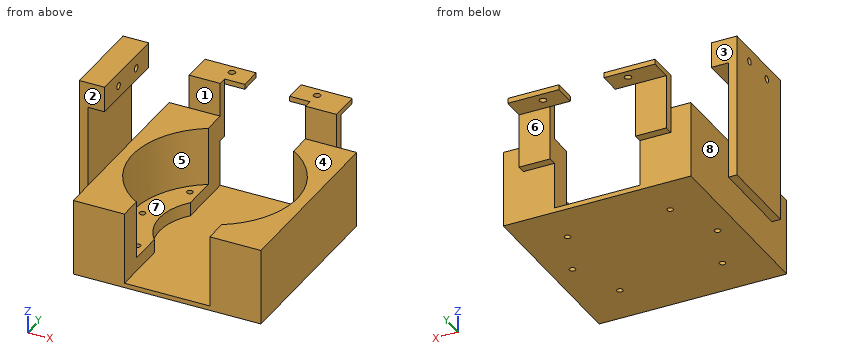
```python
from build123d import *

# Parameters (mm, degrees)
SKETCH_1_W          = 110
SKETCH_1_H          = 110
EXTRUDE_1_DEPTH     = 45
SKETCH_4_R          = 32.5
CUT_EXTRUDE_1_DEPTH = 42.3
SKETCH_5_R          = 48.25
CUT_EXTRUDE_2_DEPTH = 34.3
SKETCH_6_W          = 50
SKETCH_6_H          = 110
CUT_EXTRUDE_3_DEPTH = 8
CUT_EXTRUDE_4_DEPTH = 42.3
SKETCH_8_R          = 1.75
CUT_EXTRUDE_5_DEPTH = 160.3
SKETCH_9_W          = 18.158603558
SKETCH_9_H          = 15
SKETCH_9_H_2        = 20
EXTRUDE_2_DEPTH     = 5
SKETCH_10_W         = 30
SKETCH_10_H         = 3
EXTRUDE_3_DEPTH     = 13
SKETCH_11_R         = 2
CUT_EXTRUDE_6_DEPTH = 168.463428843
SKETCH_12_W         = 85
SKETCH_12_H         = 50
EXTRUDE_4_DEPTH     = 5
EXTRUDE_5_REACH     = 191.262
SKETCH_13_W         = 15
SKETCH_13_H         = 50
CUT_EXTRUDE_8_REACH = 194.211
SKETCH_15_RX        = 2
SKETCH_15_RY        = 1.999994073


with BuildPart() as part:
    # 草图1 → 凸台-拉伸1 (new body)
    with BuildSketch(Plane.XY):
        with Locations((55, -55)):
            Rectangle(SKETCH_1_W, SKETCH_1_H)
    extrude(amount=EXTRUDE_1_DEPTH)

    # 草图4 → 切除-拉伸1 (cut)
    with BuildSketch(Plane.XY.offset(45)):
        with Locations((55, -55)):
            Circle(SKETCH_4_R)
    extrude(amount=-CUT_EXTRUDE_1_DEPTH, mode=Mode.SUBTRACT)

    # 草图5 → 切除-拉伸2 (cut)
    with BuildSketch(Plane.XY.offset(45)):
        with Locations((55, -55)):
            Circle(SKETCH_5_R)
    extrude(amount=-CUT_EXTRUDE_2_DEPTH, mode=Mode.SUBTRACT)

    # 草图6 → 切除-拉伸3 (cut)
    with BuildSketch(Plane.XY.offset(10.7)):
        with Locations((55, -55)):
            Rectangle(SKETCH_6_W, SKETCH_6_H)
    extrude(amount=-CUT_EXTRUDE_3_DEPTH, mode=Mode.SUBTRACT)

    # 草图7 → 切除-拉伸4 (cut)
    with BuildSketch(Plane.XY.offset(45)):
        with BuildLine():
            Line((80, -34.233440343), (80, 0))
            Line((80, 0), (30, 0))
            Line((30, 0), (30, -34.233440343))
            ThreePointArc((30, -34.233440343), (22.5, -55), (30, -75.766559657))
            Line((30, -75.766559657), (30, -110))
            Line((30, -110), (80, -110))
            Line((80, -110), (80, -75.766559657))
            ThreePointArc((80, -75.766559657), (87.5, -55), (80, -34.233440343))
        make_face()
    extrude(amount=-CUT_EXTRUDE_4_DEPTH, mode=Mode.SUBTRACT)

    # 草图8 → 切除-拉伸5 (cut, through all)
    with BuildSketch(Plane.XY.offset(10.7)):
        with Locations((12.5, -55)):
            Circle(SKETCH_8_R)
        with Locations((24.9479618, -24.9479618)):
            Circle(SKETCH_8_R)
        with Locations((85.0520382, -24.9479618)):
            Circle(SKETCH_8_R)
        with Locations((97.5, -55)):
            Circle(SKETCH_8_R)
        with Locations((85.0520382, -85.0520382)):
            Circle(SKETCH_8_R)
        with Locations((24.9479618, -85.0520382)):
            Circle(SKETCH_8_R)
    extrude(amount=-CUT_EXTRUDE_5_DEPTH, mode=Mode.SUBTRACT)

    # 草图9 → 凸台-拉伸2 (add)
    with BuildSketch(Plane(origin=(0, 0, 0), x_dir=(1, 0, 0), z_dir=(0, 1, 0))):
        with Locations((20.920698221, -37.5)):
            Rectangle(SKETCH_9_W, SKETCH_9_H)
        with Locations((20.920698221, -55)):
            Rectangle(SKETCH_9_W, SKETCH_9_H_2)
        with Locations((89.079301779, -37.5)):
            Rectangle(SKETCH_9_W, SKETCH_9_H)
        with Locations((89.079301779, -55)):
            Rectangle(SKETCH_9_W, SKETCH_9_H_2)
    extrude(amount=EXTRUDE_2_DEPTH)

    # 草图10 → 凸台-拉伸3 (add)
    with BuildSketch(Plane(origin=(0, 5, 0), x_dir=(1, 0, 0), z_dir=(0, 1, 0))):
        with Locations((83.158603558, -63.5)):
            Rectangle(SKETCH_10_W, SKETCH_10_H)
        with Locations((26.841396442, -63.5)):
            Rectangle(SKETCH_10_W, SKETCH_10_H)
    extrude(amount=EXTRUDE_3_DEPTH)

    # 草图11 → 切除-拉伸6 (cut, through all)
    with BuildSketch(Plane(origin=(0, 0, 62), x_dir=(-1, 0, 0), z_dir=(0, 0, -1))):
        with Locations((-30.425668719, 12.656132332)):
            Circle(SKETCH_11_R)
        with Locations((-80.424676819, 12.34118954)):
            Circle(SKETCH_11_R)
    extrude(amount=-CUT_EXTRUDE_6_DEPTH, mode=Mode.SUBTRACT)

    # 草图12 → 凸台-拉伸4 (add)
    with BuildSketch(Plane.ZY):
        with Locations((65.296402905, -68.092997568)):
            Rectangle(SKETCH_12_W, SKETCH_12_H)
    extrude(amount=EXTRUDE_4_DEPTH)

    # 凸台-拉伸5: up to this plane
    extrude_5_end = Plane(origin=(9.859168453, -77.216105133, 215), z_dir=(-0.9999801620108199, 0.006298855833765048, 1.0454600148553557e-15))
    # 草图13 → 凸台-拉伸5 (add, up to the surface)
    with BuildSketch(Plane(origin=(0, 0, 0), x_dir=(0, 0, -1), z_dir=(1, 0, 0)), mode=Mode.PRIVATE) as extrude_5_sk1:
        with Locations((-100.296402905, -68.092997568)):
            Rectangle(SKETCH_13_W, SKETCH_13_H)
    extrude_5_tool1 = split(extrude(extrude_5_sk1.sketch, amount=EXTRUDE_5_REACH, mode=Mode.PRIVATE), bisect_by=extrude_5_end, keep=Keep.BOTH, mode=Mode.PRIVATE)
    add(extrude_5_tool1.solids().sort_by_distance((0, -68.092998, 100.296403))[0])

    # 切除-拉伸8: up to this plane
    cut_extrude_8_end = Plane(origin=(9.859168453, -77.216105133, 215), z_dir=(-0.9999801620108199, 0.006298855833765048, 1.0454600148553557e-15))
    # 草图15 → 切除-拉伸8 (cut, up to the surface)
    with BuildSketch(Plane.ZY.offset(5), mode=Mode.PRIVATE) as cut_extrude_8_sk1:
        with Locations(Location((100, -57.347927742), (0, 0, -180))):
            Ellipse(SKETCH_15_RX, SKETCH_15_RY)
    cut_extrude_8_tool1 = split(extrude(cut_extrude_8_sk1.sketch, amount=-CUT_EXTRUDE_8_REACH, mode=Mode.PRIVATE), bisect_by=cut_extrude_8_end, keep=Keep.BOTH, mode=Mode.PRIVATE)
    add(cut_extrude_8_tool1.solids().sort_by_distance((-5, -57.347928, 100))[0], mode=Mode.SUBTRACT)
    # 草图15 → 切除-拉伸8 (cut, up to the surface)
    with BuildSketch(Plane.ZY.offset(5), mode=Mode.PRIVATE) as cut_extrude_8_sk2:
        with BuildLine():
            add(Edge.make_bspline(
                [(102, -77.347868558), (102.000000089, -75.347874441), (100.000000045, -75.347874396), (98, -75.347874352), (98, -77.347868469)],
                knots=[3.141592609, 3.141592609, 3.141592609, 4.712388958, 4.712388958, 6.283185307, 6.283185307, 6.283185307], degree=2, weights=[1, 0.707106773, 1, 0.707106773, 1]))
            add(Edge.make_bspline(
                [(98, -77.347868469), (98, -79.347862497), (99.999999955, -79.347862542), (101.999999911, -79.347862586), (102, -77.347868558)],
                knots=[0, 0, 0, 1.570796304, 1.570796304, 3.141592609, 3.141592609, 3.141592609], degree=2, weights=[1, 0.707106789, 1, 0.707106789, 1]))
        make_face()
    cut_extrude_8_tool2 = split(extrude(cut_extrude_8_sk2.sketch, amount=-CUT_EXTRUDE_8_REACH, mode=Mode.PRIVATE), bisect_by=cut_extrude_8_end, keep=Keep.BOTH, mode=Mode.PRIVATE)
    add(cut_extrude_8_tool2.solids().sort_by_distance((-5, -77.347868, 100))[0], mode=Mode.SUBTRACT)


solid = part.part
```
The listing builds one solid part. Answer for the finished solid, in the listing's coordinates (mm). Face numbers are marked on the shaded views. A direction names the side the tool comes from. Coordinates: 2 decimals unless noted, no trailing zeros. Loops run counter-clockwise (first coordinate to the right, second up) from the corner with the lowest first, then second, coordinate; pieces in that order, holes last. Notation, with made-up numbers: (19.25, 41.5) - (53.25, 41.5) arc R28 cw to (53.25, 74.5) - close; hole circle Ø1 at (-21, 58.25). An arc over 180 degrees is marked (long way). Use a Markdown table: item, result. Add a question column.
1) The part is cut by section B-B, the plane x = 75. Give the vertices of the cut face in (y, z), and give its area (3 significant figures).
2) The mould has two halves that part along Y. Classify the marked faces 6, 7 and 8: released by +Y, released by -Y, zero draft, split by the parting line, or undercut.
3) The part is cut by section A-A, the plane z = 33. Give the vertices of the cut face in (x, y).
4) Given pin 1 (2 mm diameter, centred on x = 21.5, y = -9, fed in from -Z); pin 2 (0.9 mm diameter, centred on y = 12.5, z = 63, fed in from +X); pin 3 (1.5 mm diameter, centred on x = -1.5, y = -67, fed in from -Z); pin 4 (1.5 mm diameter, centred on x = 90, y = 3, fed in from -Z), each flat-ended and moving along its own axis, determine where each tip first touches the part or whether it passes through.
5) For the marked faces 1, 2, 3, 4 and 5, determine the directions among +Z, -Z, +X, -X, +Y, -Y from which every point of the face is accessible in a straight line to the end or side of a thin tool.
6) The part is cut by section C-C, the plane y = -38. Give the vertices of the cut face in (x, z).
7) Find the intervals of material crossed by line 1 (Z direction, x = 6.5, y = -77); line 2 (X direction, y = -100, z = 31); line 3 (X direction, y = -61.5, z = 5.5), in increasing order.
8) The part is cut by section D-D, the plane z = 84.5. Give the vertices of the cut face in (x, y), and give its area (3 significant figures).
Here are the results:
| question | item | result |
|---|---|---|
| 1 | outline | (-110, 0) - (0, 0) - (0, 2.7) - (-110, 2.7) - close; (5, 62) - (18, 62) - (18, 65) - (5, 65) - close |
| 1 | area | 336 mm^2 |
| 2 | face 6 | released by +Y |
| 2 | face 7 | undercut |
| 2 | face 8 | zero draft |
| 3 | outline | (-5, -93.09) - (0, -93.09) - (0, -110) - (30, -110) - (30, -96.27) arc R48.25 cw to (30, -13.73) - (30, 5) - (11.84, 5) - (11.84, 0) - (0, 0) - (0, -43.09) - (-5, -43.09) - close; (80, -110) - (110, -110) - (110, 0) - (98.16, 0) - (98.16, 5) - (80, 5) - (80, -13.73) arc R48.25 cw to (80, -96.27) - close |
| 4 | pin 1 | stops at z = 0 |
| 4 | pin 2 | stops at x = 98.16 |
| 4 | pin 3 | stops at z = 22.8 |
| 4 | pin 4 | stops at z = 30 |
| 5 | face 1 | +Z, +X, -X, -Y |
| 5 | face 2 | +Z, -X, -Y |
| 5 | face 3 | +Z, -X, +Y |
| 5 | face 4 | +Z, +X, -Y |
| 5 | face 5 | none |
| 6 | outline | (0, 0) - (110, 0) - (110, 45) - (100.16, 45) - (100.16, 10.7) - (82.7, 10.7) - (82.7, 2.7) - (27.3, 2.7) - (27.3, 10.7) - (9.84, 10.7) - (9.84, 45) - (0, 45) - close |
| 7 | line 1 | z = 0 to 45, 92.8 to 98.03, 101.97 to 107.8 |
| 7 | line 2 | x = 0 to 30, 80 to 110 |
| 7 | line 3 | x = 0 to 23.16, 86.84 to 110 |
| 8 | outline | (-5, -93.09) - (0, -93.09) - (0, -43.09) - (-5, -43.09) - close |
| 8 | area | 250 mm^2 |
